Geometry: final body of the model. Coordinates: model frame, mm. A direction names the side the tool comes from. Give positions to 0.01 mm unless a question says otherwise; leave off trailing zeros. Write each loop counter-clockwise with the first axis right and the second up, starting at its lowest first coordinate (ties: lowest second). Pieces come first, ordered by that corner, then holes.
```python
from build123d import *

# Parameters (mm, degrees)
BOSS_EXTRUDE1_DEPTH = 120.65
SKETCH2_W           = 2
SKETCH2_H           = 2.353948419


with BuildPart() as part:
    # Sketch1 → Boss-Extrude1 (new body)
    with BuildSketch(Plane(origin=(0, 0, 0), x_dir=(0, 0, -1), z_dir=(1, 0, 0))):
        Polygon((0, 7.332348419), (-6.35, 3.666174209), (-6.35, -3.666174209), (0, -7.332348419), (6.35, -3.666174209), (6.35, 3.666174209), align=None)
    extrude(amount=BOSS_EXTRUDE1_DEPTH)

    # Sketch2 → Cut-Revolve1 (revolve, cut)
    with BuildSketch(Plane.XY):
        with Locations((115.3, 6.15537421)):
            Rectangle(SKETCH2_W, SKETCH2_H)
        with Locations((14.748, 6.15537421)):
            Rectangle(SKETCH2_W, SKETCH2_H)
    revolve(axis=Axis((0, 0, 0), (1, 0, 0)), mode=Mode.SUBTRACT)


solid = part.part
```
Item 1: Section A-A, the plane x = 84.5. Return the cut outline in (y, z), plus the area to 3 significant figures.
Found:
outline: (-7.33, 0) - (-3.67, -6.35) - (3.67, -6.35) - (7.33, 0) - (3.67, 6.35) - (-3.67, 6.35) - close
area: 140 mm2
Item 2: Section B-B, the plane z = 3. Return the cut outline in (x, y), plus the area to 3 significant figures.
Found:
outline: (0, -5.6) - (13.75, -5.6) - (13.75, -3.97) - (15.75, -3.97) - (15.75, -5.6) - (114.3, -5.6) - (114.3, -3.97) - (116.3, -3.97) - (116.3, -5.6) - (120.65, -5.6) - (120.65, 5.6) - (116.3, 5.6) - (116.3, 3.97) - (114.3, 3.97) - (114.3, 5.6) - (15.75, 5.6) - (15.75, 3.97) - (13.75, 3.97) - (13.75, 5.6) - (0, 5.6) - close
area: 1,340 mm2
Item 3: Line query: L1, parallel to X at y = -3.75, z = -5.5; L2, parallel to Z at x = 94, y = -5; L3, parallel to Y at x = 58, z = -4.75. Output: solid intervals per line, ascending.
Found:
L1: x = 0 to 13.75, 15.75 to 114.3, 116.3 to 120.65
L2: z = -4.04 to 4.04
L3: y = -4.59 to 4.59
Item 4: Reachability of faces 1 (the face through (6.778, 5.474, -3.219)), 2 (the face through (114.3, -4.3, 2.9)) from +Z, -Z, +X, -X, +Y, -Y: full face, straight path, thin tool, end or side. Return the list, or none.
Found:
face 1: -Z, +X, -X, +Y
face 2: none
Item 5: Section C-C, the plane z = -3.5. Return the cut outline in (x, y).
Found:
outline: (0, -5.31) - (13.75, -5.31) - (13.75, -3.54) - (15.75, -3.54) - (15.75, -5.31) - (114.3, -5.31) - (114.3, -3.54) - (116.3, -3.54) - (116.3, -5.31) - (120.65, -5.31) - (120.65, 5.31) - (116.3, 5.31) - (116.3, 3.54) - (114.3, 3.54) - (114.3, 5.31) - (15.75, 5.31) - (15.75, 3.54) - (13.75, 3.54) - (13.75, 5.31) - (0, 5.31) - close
Item 6: Pin query (flat end, axial travel): pin 1 Ø6 at (x, z) = (21, -4) entering from +Y (3 decimals); pin 2 Ø4 at (x, z) = (107, 4.5) entering from +Y; pin 3 Ø3 at (x, z) = (54, -1) entering from -Y. Return the tip coordinate at first contact, or that it passes through.
Found:
pin 1: stops at y = 6.755
pin 2: stops at y = 5.89
pin 3: stops at y = -7.33
